Job drawing, mm, ordinate dimensions from the low corner. One solid piece. Round coordinates to 2 decimals unless told otherwise and drop trailing zeros. Loops run counter-clockwise (first coordinate to the right, second up) from the corner with the lowest first, then second, coordinate; pieces in that order, holes last. Notation, with made-up numbers: M -28,74 L 1,74 A28 ccw 1,109 Z; hole C 18,23 d4. An arc over 180 degrees is marked long. Use one line per item in the form item = value.
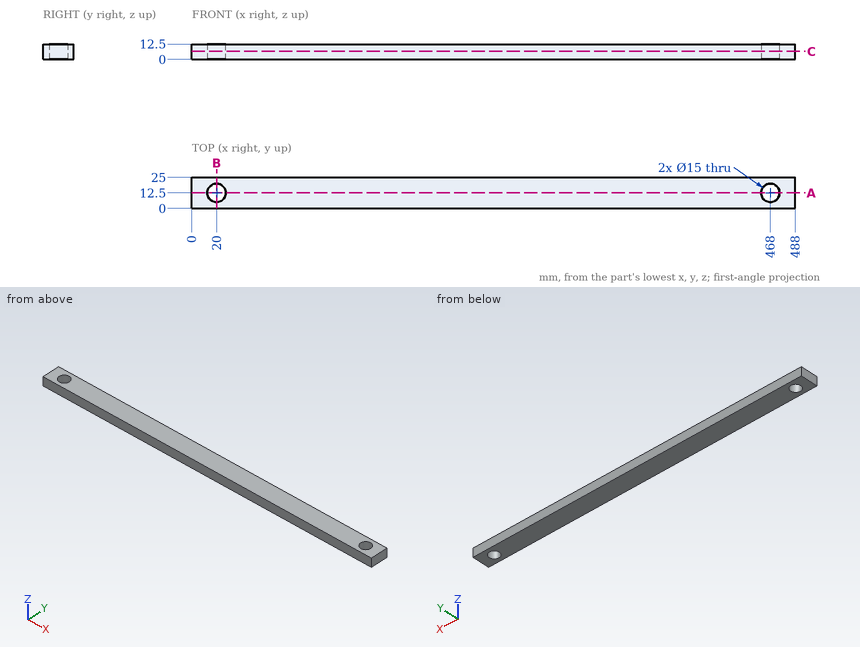
1. Probe line 1 along X through (y, z) = (12.5, 9.5); line 2 along X through (y, z) = (18, 2.75); line 3 along Y through (x, z) = (468, 5.25). List the from-to ranges inside material, lowest first. Write a range as from..to.
Completed:
line_1 = 0..12.5, 27.5..460.5, 475.5..488
line_2 = 0..14.9, 25.1..462.9, 473.1..488
line_3 = 0..5, 20..25
2. Cut at C-C on z = 6.5. Write the cut outline in (x, y).
Completed:
outline = M 0,0 L 488,0 L 488,25 L 0,25 Z; hole C 20,12.5 d15; hole C 468,12.5 d15
3. Drop a flat-ended pin along its axis: P1, Ø4, axis at x = 343.5, z = 7, coming from the -Y side. Give the stop position or say it passes through.
Completed:
P1 = 0
4. Cut at A-A on y = 12.5. Write the cut outline in (x, z).
Completed:
outline = M 0,0 L 12.5,0 L 12.5,12.5 L 0,12.5 Z; M 27.5,0 L 460.5,0 L 460.5,12.5 L 27.5,12.5 Z; M 475.5,0 L 488,0 L 488,12.5 L 475.5,12.5 Z
5. Cut at B-B on x = 20. Write the cut outline in (y, z), and give its area (3 significant figures).
Completed:
outline = M 0,0 L 5,0 L 5,12.5 L 0,12.5 Z; M 20,0 L 25,0 L 25,12.5 L 20,12.5 Z
area = 125 mm2
